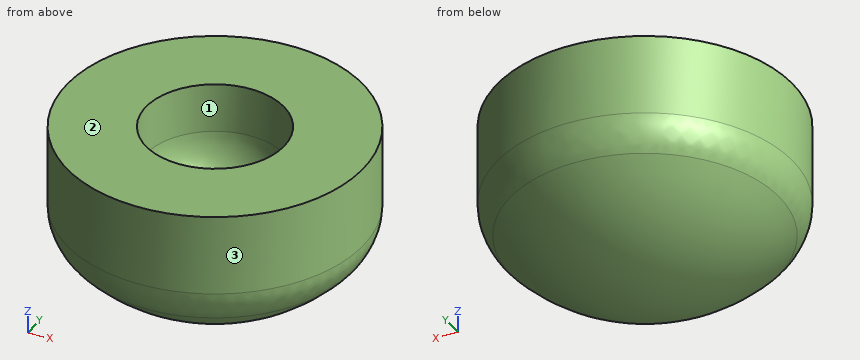
from build123d import *

# Parameters (mm, degrees)
CROQUIS1_W              = 6
CROQUIS1_H              = 8
CROQUIS1_R              = 1.4
SALIENTE_EXTRUIR1_DEPTH = 2
SALIENTE_EXTRUIR2_DEPTH = 4
CROQUIS3_W              = 6
CROQUIS3_H              = 1
SALIENTE_EXTRUIR3_DEPTH = 4
REDONDEO1_R             = 1
REDONDEO2_R             = 1


with BuildPart() as part:
    # Croquis1 → Saliente-Extruir1 (new body)
    with BuildSketch(Plane.XY):
        Rectangle(CROQUIS1_W, CROQUIS1_H)
        Circle(CROQUIS1_R, mode=Mode.SUBTRACT)
    extrude(amount=SALIENTE_EXTRUIR1_DEPTH)

    # Croquis2 → Saliente-Extruir2 (add, symmetric)
    with BuildSketch(Plane(origin=(0, 0, 0), x_dir=(1, 0, 0), z_dir=(0, 1, 0))):
        with BuildLine():
            Line((-3, 0), (3, 0))
            ThreePointArc((3, 0), (0, 1.5), (-3, 0))
        make_face()
    extrude(amount=SALIENTE_EXTRUIR2_DEPTH, both=True)

    # Croquis3 → Saliente-Extruir3 (add)
    with BuildSketch(Plane.XY.offset(2)):
        with Locations((0, 3.5)):
            Rectangle(CROQUIS3_W, CROQUIS3_H)
        with Locations((0, -3.5)):
            Rectangle(CROQUIS3_W, CROQUIS3_H)
    extrude(amount=-SALIENTE_EXTRUIR3_DEPTH)

    # Redondeo1
    redondeo1_edges = [part.edges().sort_by_distance(p)[0] for p in [
        (-1.4, 0, 0),
    ]]
    fillet(redondeo1_edges, radius=REDONDEO1_R)

    # Croquis4 → Cortar-Revolución2 (revolve, cut)
    with BuildSketch(Plane(origin=(0, 0, 0), x_dir=(0, 0, -1), z_dir=(1, 0, 0))):
        with BuildLine():
            Line((0, 3), (-2, 3))
            Line((-2, 3), (-2, 10))
            Line((-2, 10), (3, 10))
            Line((3, 10), (3, 0))
            Line((3, 0), (1.5, 0))
            ThreePointArc((1.5, 0), (1.104101966, 1.677050983), (0, 3))
        make_face()
    revolve(axis=Axis((0, 0, 2), (0, 0, -1)), mode=Mode.SUBTRACT)

    # Redondeo2
    redondeo2_edges = [part.edges().sort_by_distance(p)[0] for p in [
        (0, -3, 0),
    ]]
    fillet(redondeo2_edges, radius=REDONDEO2_R)


solid = part.part
For this review, take the finished solid that the model builds, in its own axes (mm). Face numbers are marked on the shaded views. Coordinates: 2 decimals unless noted, no trailing zeros. Order: outer loops, then holes, each group sorted by start corner. A loop starts at its lowest first (then second) coordinate and runs counter-clockwise, first axis right, second up. Notation, with made-up numbers: (-36, 66) -> (-14, 66) arc R35 ccw to (-14, 101) -> close; hole circle Ø8 at (89, 5.5). An arc over 180 degrees is marked (long way). Return JSON: item names as keys, results as strings.
1. We need section B-B on z = -1.3. Write out the cut boundary in (x, y).
Answer block:
{"outline": "circle Ø2.42 at (0, 0)"}
2. The part is to be moulded in two halves that separate along X. For the marked faces 1, 2 and 3, say which applies: +X half, -X half, draft (parallel to the pull), parting line (faces both ways), or undercut.
Answer block:
{"face 1": "undercut", "face 2": "draft", "face 3": "parting line"}
3. We need section A-A on z = 1.4. Write out the cut boundary in (x, y), and give its area (3 significant figures).
Answer block:
{"outline": "circle Ø6 at (0, 0); hole circle Ø2.8 at (0, 0)", "area": "22.1 mm²"}
4. For pin 1 Ø2 at (x, y) = (2, 1) entering from -Z; pin 2 Ø2 at (y, z) = (0.5, 1) entering from -X; pin 3 Ø1.5 at (x, y) = (2.5, 2) entering from -Z, all flat-tipped, find the tip position at first contact; note any pin that passes through.
Answer block:
{"pin 1": "z = -1.29", "pin 2": "x = -3", "pin 3": "z = -0.59"}
5. For line 1 (Y direction, x = 0, z = 1.35); line 2 (X direction, y = -0.5, z = 1.25); line 3 (Y direction, x = 1, z = 1.5), list the stretches that pass through material, from the lowest coordinate up. Write a range as from..to.
Answer block:
{"line 1": "-3..-1.4, 1.4..3", "line 2": "-2.96..-1.31, 1.31..2.96", "line 3": "-2.83..-0.98, 0.98..2.83"}
